```python
from build123d import *

# Parameters (mm, degrees)
SKETCH1_R           = 2.35
BOSS_EXTRUDE1_DEPTH = 3
FILLET1_R           = 1
FILLET2_R           = 2


with BuildPart() as part:
    # Sketch1 → Boss-Extrude1 (new body)
    with BuildSketch(Plane(origin=(0, 0, 0), x_dir=(1, 0, 0), z_dir=(0, 1, 0))):
        with BuildLine():
            Line((150.782624159, -101.436632834), (142.429643363, -95.352389557))
            ThreePointArc((142.429643363, -95.352389557), (134.417437791, -99.906414375), (136.757444533, -90.99243947))
            Line((136.757444533, -90.99243947), (133.083209919, -87.318204856))
            Line((133.083209919, -87.318204856), (134.497423481, -85.903991293))
            Line((134.497423481, -85.903991293), (97.513018177, -48.919585989))
            ThreePointArc((97.513018177, -48.919585989), (97.220124958, -48.212479208), (97.513018177, -47.505372427))
            Line((97.513018177, -47.505372427), (103.523425817, -41.494964787))
            ThreePointArc((103.523425817, -41.494964787), (104.402105474, -39.373644443), (103.523425817, -37.2523241))
            Line((103.523425817, -37.2523241), (97.159464787, -30.888363069))
            ThreePointArc((97.159464787, -30.888363069), (95.038144443, -30.009683412), (92.9168241, -30.888363069))
            Line((92.9168241, -30.888363069), (86.906416459, -36.898770709))
            ThreePointArc((86.906416459, -36.898770709), (86.199309678, -37.191663928), (85.492202897, -36.898770709))
            Line((85.492202897, -36.898770709), (58.622145212, -10.028713024))
            ThreePointArc((58.622145212, -10.028713024), (57.915038431, -9.735819805), (57.20793165, -10.028713024))
            Line((57.20793165, -10.028713024), (51.5510774, -15.685567273))
            ThreePointArc((51.5510774, -15.685567273), (51.258184181, -16.392674055), (51.5510774, -17.099780836))
            Line((51.5510774, -17.099780836), (78.421135085, -43.969838521))
            ThreePointArc((78.421135085, -43.969838521), (78.714028304, -44.676945302), (78.421135085, -45.384052083))
            Line((78.421135085, -45.384052083), (72.410727445, -51.394459723))
            ThreePointArc((72.410727445, -51.394459723), (71.532047789, -53.515780067), (72.410727445, -55.63710041))
            Line((72.410727445, -55.63710041), (78.774688476, -62.001061441))
            ThreePointArc((78.774688476, -62.001061441), (80.896008819, -62.879741098), (83.017329163, -62.001061441))
            Line((83.017329163, -62.001061441), (89.027736803, -55.990653801))
            ThreePointArc((89.027736803, -55.990653801), (89.734843584, -55.697760582), (90.441950365, -55.990653801))
            Line((90.441950365, -55.990653801), (127.426355669, -92.975059105))
            Line((127.426355669, -92.975059105), (128.840569232, -91.560845543))
            Line((128.840569232, -91.560845543), (131.668996357, -94.389272667))
            ThreePointArc((131.668996357, -94.389272667), (133.388387651, -100.345014415), (139.458762793, -101.601084408))
            Line((139.458762793, -101.601084408), (146.779034385, -106.933110699))
            ThreePointArc((146.779034385, -106.933110699), (151.529068204, -106.186666654), (150.782624159, -101.436632834))
        make_face()
        with Locations(Location((148.780829272, -104.184871767, 0), (0, 0, 270))):
            Circle(SKETCH1_R, mode=Mode.SUBTRACT)
        with BuildLine():
            Line((77.996871016, -51.323749045), (92.846113421, -36.47450664))
            ThreePointArc((92.846113421, -36.47450664), (97.937282246, -36.47450664), (97.937282246, -41.565675465))
            Line((97.937282246, -41.565675465), (83.088039841, -56.41491787))
            ThreePointArc((83.088039841, -56.41491787), (77.996871016, -56.41491787), (77.996871016, -51.323749045))
        make_face(mode=Mode.SUBTRACT)
        with BuildLine():
            Line((96.098804615, -52.455119895), (131.454143674, -87.810458954))
            ThreePointArc((131.454143674, -87.810458954), (131.454143674, -89.931779298), (129.332823331, -89.931779298))
            Line((129.332823331, -89.931779298), (93.977484271, -54.576440239))
            ThreePointArc((93.977484271, -54.576440239), (93.977484271, -52.455119895), (96.098804615, -52.455119895))
        make_face(mode=Mode.SUBTRACT)
        with BuildLine():
            Line((58.975698603, -15.332013883), (81.572324274, -37.990180363))
            ThreePointArc((81.572324274, -37.990180363), (81.572344991, -40.083780173), (79.478745181, -40.08380089))
            Line((79.478745181, -40.08380089), (56.854378259, -17.453334226))
            ThreePointArc((56.854378259, -17.453334226), (56.854378259, -15.332013883), (58.975698603, -15.332013883))
        make_face(mode=Mode.SUBTRACT)
    extrude(amount=BOSS_EXTRUDE1_DEPTH)

    # Fillet1
    fillet1_edges = [part.edges().sort_by_distance(p)[0] for p in [
        (139.458762793, 1.5, 101.601084408),
        (131.668996357, 1.5, 94.389272667),
        (133.083209919, 1.5, 87.318204856),
        (134.497423481, 1.5, 85.903991293),
        (128.840569232, 1.5, 91.560845543),
        (127.426355669, 1.5, 92.975059105),
    ]]
    fillet(fillet1_edges, radius=FILLET1_R - 0.0001)  # a hair under: the kernel refuses the full size

    # Fillet2
    fillet2_edges = [part.edges().sort_by_distance(p)[0] for p in [
        (136.757444533, 1.5, 90.99243947),
        (142.429643363, 1.5, 95.352389557),
    ]]
    fillet(fillet2_edges, radius=FILLET2_R)


solid = part.part
```
CAD build for the part. Positions are in the model's coordinates, mm. A direction names the side the tool comes from. Round coordinates to 2 decimals unless told otherwise and drop trailing zeros. Order: outer loops, then holes, each group sorted by start corner. A loop starts at its lowest first (then second) coordinate and runs counter-clockwise, first axis right, second up. Notation, with made-up numbers: (-12.75, 87) -> (0.25, 87) arc R13 ccw to (0.25, 102) -> close; hole circle Ø1 at (35.5, -37). An arc over 180 degrees is marked (long way). One line per question, with ' | ' between items.
Q1. Which spindle directions (+Z, -Z, +X, -X, +Y, -Y) get a long thin tool onto all of the face, cutting with end or side? Do faces 1 (the flat face through (108.33, 1.48, 73.88)), 2 (the flat face through (85.32, 1.48, 44)), 3 (the flat face through (89.954, 1.479, 33.851)), 4 (the cylindrical face through (71.532, 1.479, 53.483)). Say none if no direction does.
Completed:
face 1: +Z, +Y, -Y | face 2: +Y, -Y | face 3: -Z, +Y, -Y | face 4: -X, +Y, -Y
Q2. Slice it at B-B (y = 1.45). Give the number of separate pieces and of enclosed holes in the cut face, then the cut area to 3 significant figures.
Completed:
separate pieces: 1 | enclosed holes: 4 | area: 1,100 mm^2
Q3. Slice it at A-A (z = 82). Write the cut outline in (x, y), then the cut area to 3 significant figures.
Completed:
outline: (116.45, 0) -> (121.4, 0) -> (121.4, 3) -> (116.45, 3) -> close; (125.64, 0) -> (130.59, 0) -> (130.59, 3) -> (125.64, 3) -> close | area: 29.7 mm^2
Q4. Two-plate mould, pull along Z, no slides. Class faces 5 (the flat face through (64.8, 1.48, 30.35)), 6 (the flat face through (94, 0, 55)), 7 (the flat face through (75.548, 1.479, 58.775)): released by +Z, released by -Z, zero draft, split by the parting line, or undercut.
Completed:
face 5: undercut | face 6: zero draft | face 7: released by +Z
Q5. Drop flat-ended pins along their axis: pin 1 (1 mm diameter, centred on x = 95, y = 1, fed in from +Z); pin 2 (1 mm diameter, centred on x = 98, y = 2, fed in from +Z); pin 3 (5.5 mm diameter, centred on x = 148.78, z = 104.18, fed in from +Y). Give the stop position or say it passes through.
Completed:
pin 1: stops at z = 61.05 | pin 2: stops at z = 64.05 | pin 3: stops at y = 3
Q6. Probe probe 1 along X at (y, z) = (2.7, 33.5); probe 2 along X at (y, z) = (0.4, 60); probe 3 along X at (y, z) = (0.3, 45). List the from-to ranges inside material, lowest first.
Completed:
probe 1: x = 67.95 to 72.9, 77.09 to 82.09, 90.31 to 99.77 | probe 2: x = 76.77 to 85.02, 94.45 to 99.4, 103.64 to 108.59 | probe 3: x = 78.66 to 84.32, 94.5 to 100.02
